CAD build for the part. Positions are in the model's coordinates, mm. A direction names the side the tool comes from. Round coordinates to 2 decimals unless told otherwise and drop trailing zeros. Write each loop counter-clockwise with the first axis right and the second up, starting at its lowest first coordinate (ties: lowest second). Pieces come first, ordered by that corner, then holes. Notation, with made-up numbers: (65.5, 51) - (109.5, 51) arc R5 cw to (109.5, 56) - close; hole circle Ø11 at (41, 58). An arc over 180 degrees is marked (long way). Use one line per item in the form item = value. Start each with the question number.
Item 1: Band-saw the part on B-B, the plane x = -31.5. List the corners of the cut face in (y, z), and give its area (3 significant figures).
Item 2: Band-saw the part on D-D, the plane z = 4.25. List the corners of the cut face in (x, y).
Item 3: Band-saw the part on C-C, the plane y = -13. List the corners of the cut face in (x, z).
Item 4: Drill centre lines: L1, parallel to Z at x = -24, y = -10.25; L2, parallel to X at y = -11, z = 1.75; L3, parallel to Y at x = -29, z = 6.5. Where is each one in solid material? Low to high.
Item 5: Tool access for faces 1 (the cylindrical face through (-17.584, -13.634, 3.524)), 2 (the cylindrical face through (-11.68, -10.08, 0.63)): list every direction of +Z, -Z, +X, -X, +Y, -Y with a clear straight run to the whole face (end or side of a thin tool).
Item 6: Band-saw the part on A-A, the plane y = -9.5. List the corners of the cut face in (x, z).
Item 7: Pin check, flat tips, straight feed: pin 1 (3 mm diameter, centred on x = -17, y = -8, fed in from +Z); pin 2 (4 mm diameter, centred on y = -12.5, z = 5.5, fed in from -X); pin 3 (1 mm diameter, centred on x = -28.5, z = 6, fed in from +Y); pin 4 (1.5 mm diameter, centred on y = -12, z = 0.5, fed in from -X). Stop position of each tip, or through.
Item 8: Pull direction X, two halves, no side cores. Call faces 3 (the flat face through (-23, -10, 7.112)), 4 (the cylindrical face through (-34.538, -9.929, 0.626)): +X half, -X half, draft (parallel to the pull), parting line (faces both ways), or undercut.
from build123d import *

# Parameters (mm, degrees)
BOSS_EXTRUDE1_DEPTH = 1.27
SKETCH2_R           = 3.81
BOSS_EXTRUDE2_DEPTH = 4.572
SKETCH5_R           = 2.794
CUT_EXTRUDE1_DEPTH  = 24.638


with BuildPart() as part:
    # Sketch1 → Boss-Extrude1 (new body)
    with BuildSketch(Plane.XY):
        with BuildLine():
            ThreePointArc((-26.191844276, -6.037143701), (-34.535215397, -10.092878556), (-25.946396087, -13.599017422))
            ThreePointArc((-25.946396087, -13.599017422), (-22.954821865, -12.674647532), (-20.032282841, -13.798365326))
            ThreePointArc((-20.032282841, -13.798365326), (-11.677896645, -9.914450414), (-20.032282841, -6.030535502))
            ThreePointArc((-20.032282841, -6.030535502), (-23.110858628, -7.156966052), (-26.191844276, -6.037143701))
        make_face()
    boss_extrude1 = extrude(amount=BOSS_EXTRUDE1_DEPTH)

    # Sketch2 → Boss-Extrude2 (add)
    with BuildSketch(Plane.XY.offset(1.27)):
        with Locations((-16.757896645, -9.914450414)):
            Circle(SKETCH2_R)
        with Locations((-29.457889337, -9.928075423)):
            Circle(SKETCH2_R)
    extrude(amount=BOSS_EXTRUDE2_DEPTH)

    # Mirror1: Boss-Extrude1 across plane
    add(boss_extrude1.mirror(Plane.XY.offset(3.556)))

    # Sketch5 → Cut-Extrude1 (cut)
    with BuildSketch(Plane.XY.offset(7.112)):
        with Locations((-29.457889337, -9.928075423)):
            Circle(SKETCH5_R)
        with Locations((-16.757896645, -9.914450414)):
            Circle(SKETCH5_R)
    extrude(amount=-CUT_EXTRUDE1_DEPTH, mode=Mode.SUBTRACT)


solid = part.part
Determined:
q1.outline = (-14.58, 0) - (-11.83, 0) - (-11.83, 7.11) - (-14.58, 7.11) - (-14.58, 5.84) - (-13.14, 5.84) - (-13.14, 1.27) - (-14.58, 1.27) - close; (-8.02, 0) - (-5.28, 0) - (-5.28, 1.27) - (-6.71, 1.27) - (-6.71, 5.84) - (-5.28, 5.84) - (-5.28, 7.11) - (-8.02, 7.11) - close
q1.area = 25.9 mm²
q2.outline = circle Ø7.62 at (-29.46, -9.93); circle Ø7.62 at (-16.76, -9.91); hole circle Ø5.59 at (-29.46, -9.93); hole circle Ø5.59 at (-16.76, -9.91)
q3.outline = (-33.5, 0) - (-24.86, 0) - (-24.86, 1.27) - (-27.2, 1.27) - (-27.2, 5.84) - (-24.86, 5.84) - (-24.86, 7.11) - (-33.5, 7.11) - (-33.5, 5.84) - (-31.71, 5.84) - (-31.71, 1.27) - (-33.5, 1.27) - close; (-21.37, 0) - (-12.72, 0) - (-12.72, 1.27) - (-14.52, 1.27) - (-14.52, 5.84) - (-12.72, 5.84) - (-12.72, 7.11) - (-21.37, 7.11) - (-21.37, 5.84) - (-18.99, 5.84) - (-18.99, 1.27) - (-21.37, 1.27) - close
q4.L1 = 0 to 1.27, 5.84 to 7.11
q4.L2 = -33.11 to -32.04, -26.88 to -25.8, -20.41 to -19.33, -14.18 to -13.11
q4.L3 = -14.99 to -12.68, -7.17 to -4.87
q5.face_1 = none
q5.face_2 = +Z, -Z
q6.outline = (-34.52, 0) - (-32.22, 0) - (-32.22, 7.11) - (-34.52, 7.11) - (-34.52, 5.84) - (-33.24, 5.84) - (-33.24, 1.27) - (-34.52, 1.27) - close; (-26.7, 0) - (-19.52, 0) - (-19.52, 7.11) - (-26.7, 7.11) - close; (-13.99, 0) - (-11.69, 0) - (-11.69, 1.27) - (-12.97, 1.27) - (-12.97, 5.84) - (-11.69, 5.84) - (-11.69, 7.11) - (-13.99, 7.11) - close; hole (-25.67, 1.27) - (-20.55, 1.27) - (-20.55, 5.84) - (-25.67, 5.84) - close
q7.pin_1 = 7.11
q7.pin_2 = -34.5
q7.pin_3 = -4.87
q7.pin_4 = -34.36
q8.face_3 = draft
q8.face_4 = undercut
